Check sheet for the modelled part. Datum: model origin and axes. Units: mm. A direction names the side the tool comes from. Coordinates: 2 decimals unless noted, no trailing zeros. Loops run counter-clockwise (first coordinate to the right, second up) from the corner with the lowest first, then second, coordinate; pieces in that order, holes last. Notation, with made-up numbers: M -37,65.5 L -21,65.5 A27 ccw -21,92.5 Z; hole C 8.25,-38.5 d3. An arc over 180 degrees is marked long. Use CSV: the item, a comma, the result in double quotes. Start each with the question number.
(1) Go/stop test with flat-tipped pins: pin 1 Ø2 at (x, z) = (-23.5, 2.5) entering from +Y; pin 2 Ø2 at (y, z) = (-51.5, 3.5) entering from +X; pin 3 Ø1.5 at (x, z) = (-350, 1) entering from +Y. Record where each tip stops, or that it passes through.
(2) Set-up check for faces 1 (the flat face through (-373.715, -31.806, 1.972)), 2 (the flat face through (-238, 91, 0)), 3 (the flat face through (-135.6, 270.91, 1.97)), 4 (the flat face through (-371.012, 221.575, 1.972)), 5 (the flat face through (-238, 91, 4)): record each of +Z, -Z, +X, -X, +Y, -Y from which the full face is reachable in a straight line by a thin tool's end or side.
(3) Section check B-B on x = -80.5. Record the cut outline in (y, z), and give its area (3 significant figures).
(4) Draft check along Y on faces 6 (the flat face through (-113.022, 275.995, 1.972)), 7 (the flat face through (-135.82, -80.62, 1.97)), 8 (the flat face through (-252.9, -97.85, 1.97)). Enter one of: pulls with the +Y half, pulls with the -Y half, needs draft (parallel to the pull), parting line crosses it, or undercut.
(5) Scan lines: line 1 (X direction, y = 150, z = 3.75); line 2 (Y direction, x = -193, z = 2.95); line 3 (Y direction, x = -376, z = 1.75). Record each from-to range of solid material in increasing order.
(6) Section check C-C on y = -100.5. Record the cut outline in (x, z).
(7) Section check A-A on z = 0.7. Give the number of separate pieces and of enclosed holes in the cut face, and give its area (3 significant figures).
from build123d import *

# Parameters (mm, degrees)
BOSS_EXTRUDE1_DEPTH = 4
FILLET1_R           = 1


with BuildPart() as part:
    # Sketch1 → Boss-Extrude1 (new body)
    # profile 1 of 3: a face of its own
    with BuildSketch(Plane(origin=(0, 0, 0), x_dir=(0, 1, 0), z_dir=(0, 0, 1))):
        Polygon((-23.404255319, 275), (0, 0), (190, 0), (213.404255319, 275), (230, 470), (-40, 470), align=None)
        with BuildLine():
            ThreePointArc((37.9, 32.9), (40, 35), (42.1, 32.9))
            Line((42.1, 32.9), (42.1, 7.1))
            ThreePointArc((42.1, 7.1), (40, 5), (37.9, 7.1))
            Line((37.9, 7.1), (37.9, 32.9))
        make_face(mode=Mode.SUBTRACT)
        with BuildLine():
            Line((147.9, 7.1), (147.9, 32.9))
            ThreePointArc((147.9, 32.9), (150, 35), (152.1, 32.9))
            Line((152.1, 32.9), (152.1, 7.1))
            ThreePointArc((152.1, 7.1), (150, 5), (147.9, 7.1))
        make_face(mode=Mode.SUBTRACT)
    # profile 2 of 3: a face of its own
    with BuildSketch(Plane(origin=(0, 0, 0), x_dir=(0, 1, 0), z_dir=(0, 0, 1))):
        Polygon((-175, 230), (0, 0), (-23.404255319, 275), align=None)
        with BuildLine():
            ThreePointArc((-91.031422458, 127.898638669), (-93.974258564, 128.298283078), (-93.574614155, 131.241119184))
            Line((-93.574614155, 131.241119184), (-73.042233846, 146.863582462))
            ThreePointArc((-73.042233846, 146.863582462), (-70.099397741, 146.463938053), (-70.49904215, 143.521101947))
            Line((-70.49904215, 143.521101947), (-91.031422458, 127.898638669))
        make_face(mode=Mode.SUBTRACT)
    # profile 3 of 3: a face of its own
    with BuildSketch(Plane(origin=(0, 0, 0), x_dir=(0, 1, 0), z_dir=(0, 0, 1))):
        Polygon((213.404255319, 275), (190, 0), (365, 230), align=None)
        with BuildLine():
            Line((263.042233846, 146.863582462), (283.574614155, 131.241119184))
            ThreePointArc((283.574614155, 131.241119184), (283.974258564, 128.298283078), (281.031422458, 127.898638669))
            Line((281.031422458, 127.898638669), (260.49904215, 143.521101947))
            ThreePointArc((260.49904215, 143.521101947), (260.099397741, 146.463938053), (263.042233846, 146.863582462))
        make_face(mode=Mode.SUBTRACT)
    extrude(amount=BOSS_EXTRUDE1_DEPTH)

    # Fillet1
    fillet1_edges = [part.edges().sort_by_distance(p)[0] for p in [
        (-275, -23.404255319, 2),
        (-470, -40, 2),
        (-470, 230, 2),
        (-275, 213.404255319, 2),
        (-230, 365, 2),
        (0, 190, 2),
        (0, 0, 2),
        (-230, -175, 2),
    ]]
    fillet(fillet1_edges, radius=FILLET1_R)


solid = part.part
Outcome:
1,pin 1,"stops at y = 208.64"
1,pin 2,"stops at x = -66.37"
1,pin 3,"stops at y = 219.85"
2,face 1,"+Z, -Z, -Y"
2,face 2,"-Z, +X, -X, +Y, -Y"
2,face 3,"+Z, -Z"
2,face 4,"+Z, -Z, +Y"
2,face 5,"+Z, +X, -X, +Y, -Y"
3,outline,"M -61.25,0 L 251.25,0 L 251.25,4 L -61.25,4 Z"
3,area,"1,250 mm²"
4,face 6,"pulls with the +Y half"
4,face 7,"undercut"
4,face 8,"pulls with the -Y half"
5,line 1,"x = -470 to -35, -5 to 0"
5,line 2,"y = -146.85 to 336.85"
5,line 3,"y = -32 to 222"
6,outline,"M -252.11,0 L -132.09,0 L -132.09,4 L -252.11,4 Z"
7,separate pieces,"1"
7,enclosed holes,"4"
7,area,"150,000 mm²"
